from build123d import *

# Parameters (mm, degrees)
SKETCH1_R           = 165.1
SKETCH1_R_2         = 34.9885
SKETCH1_R_3         = 12.1285
BOSS_EXTRUDE1_DEPTH = 3.175
SKETCH2_R           = 2.5908
CUT_EXTRUDE1_DEPTH  = 6.35


with BuildPart() as part:
    # Sketch1 → Boss-Extrude1 (new, symmetric)
    with BuildSketch(Plane.XY):
        Circle(SKETCH1_R)
        with Locations((0, 114.3)):
            Circle(SKETCH1_R_2, mode=Mode.SUBTRACT)
        with Locations((98.986703653, 57.15)):
            Circle(SKETCH1_R_2, mode=Mode.SUBTRACT)
        with Locations((98.986703653, -57.15)):
            Circle(SKETCH1_R_2, mode=Mode.SUBTRACT)
        with Locations((0, -114.3)):
            Circle(SKETCH1_R_2, mode=Mode.SUBTRACT)
        with Locations((-98.986703653, -57.15)):
            Circle(SKETCH1_R_2, mode=Mode.SUBTRACT)
        with Locations((-98.986703653, 57.15)):
            Circle(SKETCH1_R_2, mode=Mode.SUBTRACT)
        Circle(SKETCH1_R_3, mode=Mode.SUBTRACT)
    extrude(amount=BOSS_EXTRUDE1_DEPTH, both=True)

    # Sketch2 → Cut-Extrude1 (cut)
    with BuildSketch(Plane(origin=(0, 0, -3.175), x_dir=(-1, 0, 0), z_dir=(0, 0, -1))):
        with Locations((-23.8125, 0)):
            Circle(SKETCH2_R)
        with Locations((-11.90625, 20.622229928)):
            Circle(SKETCH2_R)
        with Locations((11.90625, 20.622229928)):
            Circle(SKETCH2_R)
        with Locations((23.8125, 0)):
            Circle(SKETCH2_R)
        with Locations((11.90625, -20.622229928)):
            Circle(SKETCH2_R)
        with Locations((-11.90625, -20.622229928)):
            Circle(SKETCH2_R)
    extrude(amount=-CUT_EXTRUDE1_DEPTH, mode=Mode.SUBTRACT)


solid = part.part
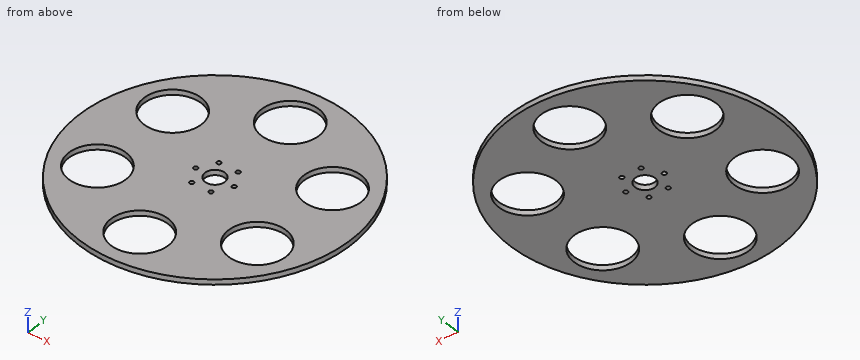
Input: part model. Units: mm. Frame: model coordinates. Coordinates: 2 decimals unless noted, no trailing zeros. Order: outer loops, then holes, each group sorted by start corner. A loop starts at its lowest first (then second) coordinate and runs counter-clockwise, first axis right, second up.
1. Cut plane B-B, the plane y = 114.3. Return loops of the section in (x, z) (1 decimal), plus the area to 3 significant figures.
Checked values:
outline: (-119.1, -3.2) - (-35, -3.2) - (-35, 3.2) - (-119.1, 3.2) - close; (35, -3.2) - (119.1, -3.2) - (119.1, 3.2) - (35, 3.2) - close
area: 1,070 mm2
2. Cut plane D-D, the plane x = 75.5. Return loops of the section in (y, z) (3 decimals).
Checked values:
outline: (-146.826, -3.175) - (-83.084, -3.175) - (-83.084, 3.175) - (-146.826, 3.175) - close; (-31.216, -3.175) - (31.216, -3.175) - (31.216, 3.175) - (-31.216, 3.175) - close; (83.084, -3.175) - (146.826, -3.175) - (146.826, 3.175) - (83.084, 3.175) - close
3. Cut plane C-C, the plane z = 0.25. Count the separate pieces of the cut face and the enclosed holes in it, plus the area to 3 significant figures.
Checked values:
separate pieces: 1
enclosed holes: 13
area: 62,000 mm2
4. Ray query, line 1 along Y through (x, z) = (0, 0.5); line 2 along Y through (x, z) = (-73, 0.75); line 3 along X through (y, z) = (84, -2). Return the intervals inside material, ascending.
Checked values:
line 1: y = -165.1 to -149.29, -79.31 to -12.13, 12.13 to 79.31, 149.29 to 165.1
line 2: y = -148.08 to -80.58, -33.72 to 33.72, 80.58 to 148.08
line 3: x = -142.13 to -121.42, -76.55 to -17.5, 17.5 to 76.55, 121.42 to 142.13
5. Contact query for flat-ended pins moving along their axis: P1, Ø8.5, axis at x = -11.91, y = 20.62, coming from the -Z side (3 decimals); P2, Ø2, axis at y = 110, z = 1, coming from the -X side; P3, Ø2, axis at y = 41, z = -1.5, coming from the -X side; P4, Ø1, axis at x = 59, z = 1, coming from the +Y side. Output: stop coordinate, or through.
Checked values:
P1: stops at z = -3.175
P2: stops at x = -124
P3: stops at x = -160.18
P4: stops at y = 154.39
6. Cut plane A-A, the plane x = 0. Return loops of the section in (y, z) (1 decimal).
Checked values:
outline: (-165.1, -3.2) - (-149.3, -3.2) - (-149.3, 3.2) - (-165.1, 3.2) - close; (-79.3, -3.2) - (-12.1, -3.2) - (-12.1, 3.2) - (-79.3, 3.2) - close; (12.1, -3.2) - (79.3, -3.2) - (79.3, 3.2) - (12.1, 3.2) - close; (149.3, -3.2) - (165.1, -3.2) - (165.1, 3.2) - (149.3, 3.2) - close
